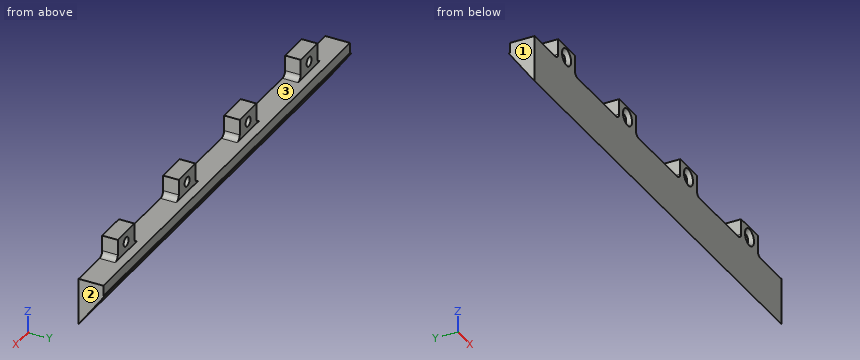
Autodesk Inventor part; units mm, degrees
ref_plane "YZ Plane" through (0, 0, 0) normal (1, 0, 0) x (0, 1, 0)
ref_plane "XZ Plane" through (0, 0, 0) normal (0, 1, 0) x (-1, 0, 0)
ref_plane "XY Plane" through (0, 0, 0) normal (0, 0, 1) x (1, 0, 0)
sketch "Sketch3" plane through (0, 0, 0) normal (1, 0, 0) x (0, 1, 0)
  line L0 (0, 0) -> (10, 0)
  line L1 (10, 0) -> (10, -14)
  line L2 (10, -14) -> (0, -14)
  line L3 (0, -14) -> (0, 0)
  line L4 (10, 0) -> (0, -14)
  line L5 (6, 0) -> (0, 0)
  line L6 (0, 0) -> (0, 12)
  line L7 (0, 12) -> (6, 12)
  line L8 (6, 12) -> (6, 0)
  line L9 (9.5, 0) -> (6, 0)
  line L10 (6, 0) -> (6, 4)
  line L11 (6, 4) -> (9.5, 4)
  line L12 (9.5, 4) -> (9.5, 0)
  dimension "d30" = 12
  dimension "d31" = 6
  dimension "d63" = 10
  dimension "d74" = 0.5
  dimension "d75" = 4
  dimension "d76" = 3.5
  dimension "d141" = 35.538
  dimension "d142" = 14
extrude "Extrusion2" add sketch "Sketch3" along normal blind 178 contours L6 L7 L8 L0 | L0 L4 L3 | L8 L11 L12 L0
sketch "Sketch10" plane through (0, 0, -14) normal (0, -1, 0) x (1, 0, 0)
  line L0 (0, 18) -> (0, 26)
  line L1 (0, 26) -> (178, 26)
  line L2 (178, 18) -> (178, 26)
  line L3 (0, 18) -> (178, 18)
  line L4 (0, 14) -> (0, 18)
  line L5 (0, 18) -> (17, 18)
  line L6 (17, 18) -> (17, 26)
  line L7 (17, 26) -> (0, 26)
  line L8 (0, 26) -> (0, 18)
  line L9 (0, 18) -> (178, 18)
  line L10 (178, 26) -> (161, 26)
  line L11 (161, 26) -> (161, 18)
  line L12 (161, 18) -> (178, 18)
  line L13 (178, 18) -> (178, 26)
  line L14 (17, 26) -> (29, 26)
  line L15 (29, 26) -> (29, 18)
  line L16 (29, 18) -> (17, 18)
  line L17 (17, 18) -> (17, 26)
  line L18 (61, 26) -> (73, 26)
  line L19 (73, 26) -> (73, 18)
  line L20 (73, 18) -> (61, 18)
  line L21 (61, 18) -> (61, 26)
  line L22 (105, 26) -> (117, 26)
  line L23 (117, 26) -> (117, 18)
  line L24 (117, 18) -> (105, 18)
  line L25 (105, 18) -> (105, 26)
  line L26 (149, 26) -> (161, 26)
  line L27 (161, 26) -> (161, 18)
  line L28 (161, 18) -> (149, 18)
  line L29 (149, 18) -> (149, 26)
  line L30 (17, 26) -> (29, 18)
  line L31 (29, 26) -> (17, 18)
  line L32 (61, 26) -> (73, 18)
  line L33 (73, 26) -> (61, 18)
  line L34 (105, 26) -> (117, 18)
  line L35 (117, 26) -> (105, 18)
  line L36 (149, 26) -> (161, 18)
  line L37 (161, 26) -> (149, 18)
  point P0 (105, 18)
  point P1 (23, 22)
  point P2 (67, 22)
  point P3 (111, 22)
  point P4 (155, 22)
  dimension "d118" = 17
  dimension "d119" = 17
  dimension "d120" = 12
  dimension "d121" = 12
  dimension "d122" = 12
  dimension "d123" = 12
  dimension "d124" = 0
  dimension "d125" = 0
  dimension "d126" = 32
  dimension "d129" = 32
  dimension "d130" = 32
extrude "Extrusion5" cut sketch "Sketch10" against normal up to next contours L0 L1 L6 L3 | L15 L1 L21 L3 | L19 L1 L25 L3 | L23 L1 L29 L3 | L11 L1 L2 L3
hole "Hole4" at (23, 0, 8) at (67, 0, 8) at (111, 0, 8) at (155, 0, 8) direction (0, 1, 0) diameter 3.6 end through all countersink diameter 6.5 countersink angle 90
fillet "Fillet2" radius 2 8 edges at (17, 3, 4) (29, 3, 4) (61, 3, 4) (73, 3, 4) (105, 3, 4) (117, 3, 4) (149, 3, 4) (161, 3, 4)
equation "\"d126\" = d130"
equation "\"d129\" = d130"
properties part number "plog" material "Steel, Alloy"
Verification items for the finished model (mm, model axes). Face numbers are marked on the shaded views. Give positions to 0.01 mm unless a question says otherwise; leave off trailing zeros. Loops run counter-clockwise (first coordinate to the right, second up) from the corner with the lowest first, then second, coordinate; pieces in that order, holes last.
1. Section check A-A, the plane x = 67. Enter the section's corners in (y, z), then the cut area to 3 significant figures.
2. Section check D-D, the plane z = -3.25. Enter the section's corners in (x, y).
3. Thickness scan on line 1 (X direction, y = 3.75, z = 11.25); line 2 (Z direction, x = 155, y = 2.85); line 3 (Z direction, x = 23, y = 3.8). Record the ranges inside material, lowest first.
4. Section check C-C, the plane x = 123.5. Enter the section's corners in (y, z), then the cut area to 3 significant figures.
5. Go/stop test with flat-tipped pins: pin 1 Ø9 at (x, z) = (69.5, 9.5) entering from +Y; pin 2 Ø1.8 at (y, z) = (3.5, 10.5) entering from -X; pin 3 Ø5 at (x, y) = (60, 3.5) entering from +Z; pin 4 Ø9 at (x, z) = (110.5, 7) entering from +Y. Record where each tip stops, or that it passes through.
6. Section check B-B, the plane y = 3.5. Count the separate pieces of the cut face and the enclosed holes in it, then the cut area to 3 significant figures.
7. Mould release check, pull along X, two halves, no side actions. Record for the marked faces 1, 2 and 3: released by +X, released by -X, zero draft, split by the parting line, or undercut.
Geometry says:
1. outline: (0, -14) - (10, 0) - (9.5, 0) - (9.5, 4) - (6, 4) - (6, 6.2) - (1.45, 6.2) - (0, 4.75) - close; (0, 11.25) - (1.45, 9.8) - (6, 9.8) - (6, 12) - (0, 12) - close
1. area: 132 mm2
2. outline: (0, 0) - (178, 0) - (178, 7.68) - (0, 7.68) - close
3. line 1: x = 17 to 29, 61 to 73, 105 to 117, 149 to 161
3. line 2: z = -10.01 to 6.2, 9.8 to 12
3. line 3: z = -8.68 to 6.2, 9.8 to 12
4. outline: (0, -14) - (10, 0) - (9.5, 0) - (9.5, 4) - (0, 4) - close
4. area: 108 mm2
5. pin 1: stops at y = 6
5. pin 2: stops at x = 17
5. pin 3: stops at z = 12
5. pin 4: stops at y = 9.5
6. separate pieces: 1
6. enclosed holes: 4
6. area: 2,680 mm2
7. face 1: released by -X
7. face 2: released by +X
7. face 3: undercut
